```python
from build123d import *

# Parameters (mm, degrees)
SKETCH4_W            = 40
SKETCH4_H            = 80
BOSS_EXTRUDE4_DEPTH  = 5
SKETCH5_W            = 10
SKETCH5_H            = 5
BOSS_EXTRUDE6_DEPTH  = 50
SKETCH7_W            = 10
SKETCH7_H            = 25
SKETCH7_H_2          = 5
BOSS_EXTRUDE7_DEPTH  = 20
SKETCH9_W            = 80
SKETCH9_H            = 5
BOSS_EXTRUDE9_DEPTH  = 10
SKETCH10_W           = 50
SKETCH10_H           = 5
BOSS_EXTRUDE10_DEPTH = 20
SKETCH11_R           = 2.25
CUT_EXTRUDE1_DEPTH   = 25
SKETCH12_R           = 4
SKETCH12_R_2         = 2.25
CUT_EXTRUDE2_DEPTH   = 2
SKETCH15_W           = 7
SKETCH15_H           = 30
BOSS_EXTRUDE11_DEPTH = 20
CUT_EXTRUDE4_REACH   = 89.464
SKETCH16_R           = 2.75
FILLET3_R            = 3
SKETCH19_W           = 7
SKETCH19_H           = 30
BOSS_EXTRUDE12_DEPTH = 5
FILLET4_R            = 2
BOSS_EXTRUDE13_START = 2
SKETCH20_R           = 4
SKETCH20_R_2         = 2.25
BOSS_EXTRUDE13_DEPTH = 2


with BuildPart() as part:
    # Sketch4 → Boss-Extrude4 (new body)
    with BuildSketch(Plane(origin=(0, 0, 0), x_dir=(1, 0, 0), z_dir=(0, 1, 0))):
        with Locations((20, 40)):
            Rectangle(SKETCH4_W, SKETCH4_H)
    extrude(amount=BOSS_EXTRUDE4_DEPTH)

    # Sketch5 → Boss-Extrude6 (add)
    with BuildSketch(Plane(origin=(0, 5, 0), x_dir=(1, 0, 0), z_dir=(0, 1, 0))):
        with Locations((35, 52.5)):
            Rectangle(SKETCH5_W, SKETCH5_H)
        with Locations((35, 27.5)):
            Rectangle(SKETCH5_W, SKETCH5_H)
    extrude(amount=BOSS_EXTRUDE6_DEPTH)

    # Sketch7 → Boss-Extrude7 (add)
    with BuildSketch(Plane.XY.offset(-50)):
        with Locations((35, 17.5)):
            Rectangle(SKETCH7_W, SKETCH7_H)
        with Locations((35, 52.5)):
            Rectangle(SKETCH7_W, SKETCH7_H_2)
    extrude(amount=BOSS_EXTRUDE7_DEPTH)

    # Sketch9 → Boss-Extrude9 (add)
    with BuildSketch(Plane.ZY):
        with Locations((-40, 2.5)):
            Rectangle(SKETCH9_W, SKETCH9_H)
    extrude(amount=BOSS_EXTRUDE9_DEPTH)

    # Sketch10 → Boss-Extrude10 (add)
    with BuildSketch(Plane.XY):
        with Locations((15, 2.5)):
            Rectangle(SKETCH10_W, SKETCH10_H)
    extrude(amount=BOSS_EXTRUDE10_DEPTH)

    # Sketch11 → Cut-Extrude1 (cut, symmetric)
    with BuildSketch(Plane.XY.offset(-50)):
        with Locations((35, 40)):
            Circle(SKETCH11_R)
    extrude(amount=CUT_EXTRUDE1_DEPTH, both=True, mode=Mode.SUBTRACT)

    # Sketch12 → Cut-Extrude2 (cut)
    with BuildSketch(Plane.XY.offset(-25)):
        with Locations((35, 40)):
            Circle(SKETCH12_R)
        with Locations((35, 40)):
            Circle(SKETCH12_R_2, mode=Mode.SUBTRACT)
    extrude(amount=-CUT_EXTRUDE2_DEPTH, mode=Mode.SUBTRACT)

    # Sketch15 → Boss-Extrude11 (add)
    with BuildSketch(Plane.ZY.offset(-30)):
        with Locations((-51.5, 40)):
            Rectangle(SKETCH15_W, SKETCH15_H)
        with Locations((-28.5, 40)):
            Rectangle(SKETCH15_W, SKETCH15_H)
    extrude(amount=BOSS_EXTRUDE11_DEPTH)

    # Cut-Extrude4: up to this face of the body (flat: up to its plane)
    cut_extrude4_end = Plane(part.part.faces().sort_by_distance((26.698149798, 35.387860999, -55))[0])
    # Sketch16 → Cut-Extrude4 (cut, up to the picked face)
    with BuildSketch(Plane.XY.offset(-25), mode=Mode.PRIVATE) as cut_extrude4_sk1:
        with Locations((17, 40)):
            Circle(SKETCH16_R)
    cut_extrude4_tool1 = split(extrude(cut_extrude4_sk1.sketch, amount=-CUT_EXTRUDE4_REACH, mode=Mode.PRIVATE), bisect_by=cut_extrude4_end, keep=Keep.BOTH, mode=Mode.PRIVATE)
    add(cut_extrude4_tool1.solids().sort_by(Axis((17, 40, -25), (0, 0, -1)))[0], mode=Mode.SUBTRACT)

    # Fillet3
    fillet3_edges = [part.edges().sort_by_distance(p)[0] for p in [
        (40, 55, -40),
        (-10, 2.5, -80),
        (40, 2.5, -80),
        (-10, 2.5, 20),
        (40, 2.5, 20),
    ]]
    fillet(fillet3_edges, radius=FILLET3_R)

    # Sketch19 → Boss-Extrude12 (add)
    with BuildSketch(Plane.ZY.offset(-10)):
        with Locations((-51.5, 40)):
            Rectangle(SKETCH19_W, SKETCH19_H)
        with Locations((-28.5, 40)):
            Rectangle(SKETCH19_W, SKETCH19_H)
    extrude(amount=BOSS_EXTRUDE12_DEPTH)

    # Fillet4
    fillet4_edges = [part.edges().sort_by_distance(p)[0] for p in [
        (30, 25, -51.5),
        (30, 25, -28.5),
        (35, 5, -55),
        (30, 5, -40),
        (5, 55, -51.5),
        (5, 25, -51.5),
        (5, 25, -28.5),
        (5, 55, -28.5),
        (35, 5, -25),
    ]]
    fillet(fillet4_edges, radius=FILLET4_R)

    # Sketch20 → Boss-Extrude13 (add)
    with BuildSketch(Plane.XY.offset(-27).offset(BOSS_EXTRUDE13_START)):
        with Locations((35, 40)):
            Circle(SKETCH20_R)
        with Locations((35, 40)):
            Circle(SKETCH20_R_2, mode=Mode.SUBTRACT)
    extrude(amount=-BOSS_EXTRUDE13_DEPTH)


solid = part.part
```
The listing builds one solid part. Answer for the finished solid, in the listing's coordinates (mm). A direction names the side the tool comes from. Coordinates: 2 decimals unless noted, no trailing zeros. Write each loop counter-clockwise with the first axis right and the second up, starting at its lowest first coordinate (ties: lowest second). Pieces come first, ordered by that corner, then holes. Notation, with made-up numbers: (66, 89.25) - (118, 89.25) arc R11 ccw to (118, 97.25) - close; hole circle Ø4 at (-24.5, -17.75). An arc over 180 degrees is marked (long way). Return JSON: item names as keys, results as strings. Group by question number.
1. Straight lines are drawn through the part: L1, parallel to Y at x = 17, z = -30; L2, parallel to Y at x = 20.5, z = -51; L3, parallel to Z at x = 26, y = 36.5. For each, find the intervals that lie inside material, in ascending order.
2. A cutting plane is placed at C-C, the plane z = -43. Determine the outline of the cut face in (x, y), plus the area to 3 significant figures.
3. A cutting plane is placed at D-D, the plane y = 46. Determine the outline of the cut face in (x, z), plus the area to 3 significant figures.
4. Which of the six approach directions +Z, -Z, +X, -X, +Y, -Y give full straight-line access (tool end or side, diameter ignored) to faces 5 (the flat face through (40, 16, -37)), 6 (the cylindrical face through (29.4, 24.43, -28.45)), 7 (the flat face through (22, 37, -25)), 8 (the flat face through (20, 42, -32)), 9 (the flat face through (30, 40, -31))?
5. Given pin 1 (11 mm diameter, centred on x = 33.5, y = 42, fed in from +Z); pin 2 (18.5 mm diameter, centred on y = 21.5, z = -40.5, fed in from -X); pin 3 (12 mm diameter, centred on x = 31, y = 38.5, fed in from -Z), each flat-ended and moving along its own axis, determine where each tip first touches the part or whether it passes through.
6. A cutting plane is placed at A-A, the plane y = 40. Determine the outline of the cut face in (x, z).
7. Determine the mould class of faces 1 (the cylindrical face through (36.21, 41.897, -52.465)), 2 (the cylindrical face through (39.14, 2.54, 19.1)), 3 (the cylindrical face through (5.6, 25.57, -51.45)), 4 (the flat face through (15, 0, -31)) for opening direction Y: released by +Y, released by -Y, zero draft, split by the parting line, or undercut.
8. A cutting plane is placed at B-B, the plane x = 35. Determine the outline of the cut face in (y, z), plus the area to 3 significant figures.
Ans:
{
 "1": {"L1": "0 to 5, 25 to 37.25, 42.75 to 55", "L2": "0 to 5, 25 to 55", "L3": "-55 to -48, -32 to -25"},
 "2": {"outline": "(-10, 0) - (40, 0) - (40, 30) - (30, 30) - (30, 7) arc R2 cw to (28, 5) - (-10, 5) - close; (30, 50) - (40, 50) - (40, 52) arc R3 ccw to (37, 55) - (30, 55) - close", "area": "549 mm²"},
 "3": {"outline": "(5, -55) - (40, -55) - (40, -50) - (30, -50) - (30, -48) - (5, -48) - close; (5, -32) - (30, -32) - (30, -30) - (40, -30) - (40, -25) - (5, -25) - close", "area": "450 mm²"},
 "4": {"face 5": "+Z, -Z, +X, +Y, -Y", "face 6": "+Z, -Z, -X", "face 7": "+Z, +X, -X, +Y", "face 8": "-X, +Y", "face 9": "+X"},
 "5": {"pin 1": "z = -25", "pin 2": "x = 5", "pin 3": "z = -55"},
 "6": {"outline": "(5, -55) - (14.25, -55) - (14.25, -48) - (5, -48) - close; (5, -32) - (14.25, -32) - (14.25, -25) - (5, -25) - close; (19.75, -55) - (32.75, -55) - (32.75, -50) - (30, -50) - (30, -48) - (19.75, -48) - close; (19.75, -32) - (30, -32) - (30, -30) - (32.75, -30) - (32.75, -25) - (19.75, -25) - close; (37.25, -55) - (40, -55) - (40, -50) - (37.25, -50) - close; (37.25, -30) - (40, -30) - (40, -25) - (37.25, -25) - close"},
 "7": {"face 1": "undercut", "face 2": "zero draft", "face 3": "undercut", "face 4": "released by -Y"},
 "8": {"outline": "(0, -80) - (5, -80) - (5, -57) arc R2 cw to (7, -55) - (37.75, -55) - (37.75, -50) - (30, -50) - (30, -30) - (37.75, -30) - (37.75, -25) - (7, -25) arc R2 cw to (5, -23) - (5, 20) - (0, 20) - close; (42.25, -55) - (55, -55) - (55, -25) - (42.25, -25) - (42.25, -30) - (50, -30) - (50, -50) - (42.25, -50) - close", "area": "1,560 mm²"}
}
